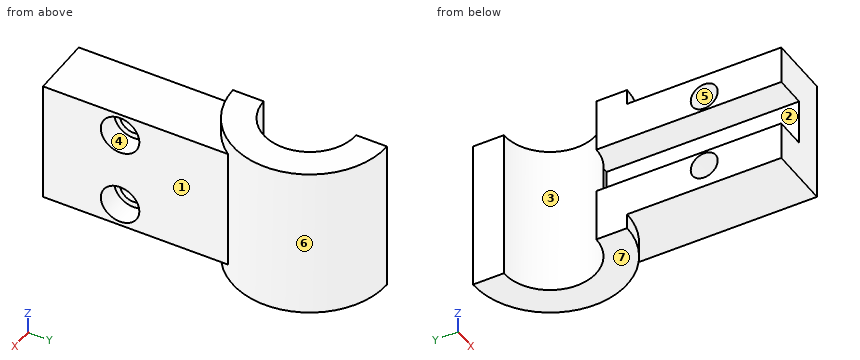
```python
from build123d import *

# Parameters (mm, degrees)
F1_DEPTH = 4
F2_DEPTH = 5
F3_W     = 12
F3_H     = 3
F3_W_2   = 0.4951214439
F4_DEPTH = 2
F5_R     = 1.25
F5_R_2   = 0.875
F6_DEPTH = 1.5
F7_DEPTH = 25


with BuildPart() as f1:
    # F0 (on Top) → F1 (new body, symmetric)
    with BuildSketch(Plane.XY):
        with BuildLine():
            Line((-2.528, 23.2174559587), (1.472, 23.2174559587))
            Line((1.472, 23.2174559587), (1.472, 35.2174559587))
            ThreePointArc((1.472, 35.2174559587), (-0.2919320225, 33.7453200037), (-2.528, 33.2174559587))
            Line((-2.528, 33.2174559587), (-2.528, 23.2174559587))
        make_face()
    extrude(amount=F1_DEPTH, both=True)

    # F0 (on Top) → F2 (join, symmetric)
    with BuildSketch(Plane.XY):
        with BuildLine():
            ThreePointArc((-2.528, 33.2174559587), (-0.2919320225, 33.7453200037), (1.472, 35.2174559587))
            ThreePointArc((1.472, 35.2174559587), (1.944135955, 40.4535239362), (-2.528, 43.2174559587))
            Line((-2.528, 43.2174559587), (-2.528, 41.2174559587))
            ThreePointArc((-2.528, 41.2174559587), (0.472, 38.2174559587), (-2.528, 35.2174559587))
            Line((-2.528, 35.2174559587), (-2.528, 33.2174559587))
        make_face()
    extrude(amount=F2_DEPTH, both=True)

    # F3 (on face) → F4 (cut)
    with BuildSketch(Plane(origin=(-2.528, 0, 0), x_dir=(0, -1, 0), z_dir=(-1, 0, 0))):
        with Locations((-29.2174559587, 0)):
            Rectangle(F3_W, F3_H)
        with Locations((-35.4650166806, 0)):
            Rectangle(F3_W_2, F3_H)
    extrude(amount=-F4_DEPTH, mode=Mode.SUBTRACT)

    # F5 (on face) → F6 (cut)
    with BuildSketch(Plane.YZ.offset(1.472)):
        with Locations((28.2174559587, 2.5)):
            Circle(F5_R)
        with Locations((28.2174559587, 2.5)):
            Circle(F5_R_2, mode=Mode.SUBTRACT)
        with Locations((28.2174559587, -2.5)):
            Circle(F5_R)
        with Locations((28.2174559587, -2.5)):
            Circle(F5_R_2, mode=Mode.SUBTRACT)
    extrude(amount=-F6_DEPTH, mode=Mode.SUBTRACT)

    # F7 (cut): faces of the model
    f7_faces = [f1.faces().sort_by_distance(p)[0] for p in [
        (1.472, 28.2174559587, 2.5),
        (1.472, 28.2174559587, -2.5),
    ]]
    extrude(f7_faces, amount=-F7_DEPTH, mode=Mode.SUBTRACT)


solid = f1.part
```
Part model, mm, in its own coordinate system. Face numbers are marked on the shaded views. A direction names the side the tool comes from. Coordinates: 2 decimals unless noted, no trailing zeros. Order: outer loops, then holes, each group sorted by start corner. A loop starts at its lowest first (then second) coordinate and runs counter-clockwise, first axis right, second up. Notation, with made-up numbers: (63.25, 4) - (80.25, 4) arc R18 cw to (80.25, 18) - close; hole circle Ø10 at (56.5, -14). An arc over 180 degrees is marked (long way). Return JSON: item names as keys, results as strings. Group by question number.
Item 1: Cut at B-B (x = -0.3). List the corners of the cut face in (y, z) (3 decimals).
Item 2: Pin check, flat tips, straight feed: pin 1 (0.9 mm diameter, centred on y = 32.5, z = -0.5, fed in from -X); pin 2 (1.2 mm diameter, centred on x = 0.5, y = 27.5, fed in from +Z); pin 3 (2 mm diameter, centred on x = 1.5, z = -0.5, fed in from +Y). Stop position of each tip, or through.
Item 3: Cut at D-D (x = 1.25). List the corners of the cut face in (y, z), plus the area to 3 significant figures.
Item 4: Cut at A-A (z = 2.5). List the corners of the cut face in (x, y).
Item 5: Pull direction Z, two halves, no side cores. Call the marked faces 5, 6 and 7: pulls with the +Z half, pulls with the -Z half, needs draft (parallel to the pull), parting line crosses it, or undercut.
Item 6: Which spindle directions (+Z, -Z, +X, -X, +Y, -Y) get a long thin tool onto all of the face, cutting with end or side? Do the marked faces 1, 2, 3 and 4. Say none if no direction does.
Item 7: Drill centre lines: probe 1 along Z at (x, y) = (-0.9, 31.25); probe 2 along Y at (x, z) = (-1.65, 3); probe 3 along Y at (x, z) = (-0.1, -3.25). Where is each one in solid material? Low to high. Write a range as from..to.
Item 8: Cut at C-C (z = 1). List the corners of the cut face in (x, y), plus the area to 3 significant figures.
Check values:
{
 "1": {"outline": "(23.217, -4) - (33.741, -4) - (33.741, -5) - (36.208, -5) - (36.208, 5) - (33.741, 5) - (33.741, 4) - (23.217, 4) - close; (40.226, -5) - (42.694, -5) - (42.694, 5) - (40.226, 5) - close; hole circle Ø1.75 at (28.217, -2.5); hole circle Ø1.75 at (28.217, 2.5)"},
 "2": {"pin 1": "stops at x = -0.53", "pin 2": "stops at z = 4", "pin 3": "stops at y = 42.2"},
 "3": {"outline": "(23.22, -4) - (34.94, -4) - (34.94, -5) - (41.49, -5) - (41.49, 5) - (34.94, 5) - (34.94, 4) - (23.22, 4) - close; hole circle Ø2.5 at (28.22, -2.5); hole circle Ø2.5 at (28.22, 2.5)", "area": "149 mm2"},
 "4": {"outline": "(-2.53, 23.22) - (1.47, 23.22) - (1.47, 26.97) - (-0.03, 26.97) - (-0.03, 27.34) - (-2.53, 27.34) - close; (-2.53, 29.09) - (-0.03, 29.09) - (-0.03, 29.47) - (1.47, 29.47) - (1.47, 35.22) arc R5 ccw to (-2.53, 43.22) - (-2.53, 41.22) arc R3 cw to (-2.53, 35.22) - close"},
 "5": {"face 5": "undercut", "face 6": "needs draft", "face 7": "pulls with the -Z half"},
 "6": {"face 1": "+Z, -Z, +X, -Y", "face 2": "-X, -Y", "face 3": "+Z, -Z, -X", "face 4": "+X"},
 "7": {"probe 1": "z = -4..-1.5, 1.5..4", "probe 2": "y = 23.22..27.5, 28.94..35.35, 41.09..43.14", "probe 3": "y = 23.22..27.77, 28.67..36.46, 39.98..42.59"},
 "8": {"outline": "(-2.53, 41.22) arc R3 cw to (-0.88, 35.71) - (-0.53, 35.71) - (-0.53, 23.22) - (1.47, 23.22) - (1.47, 35.22) arc R5 ccw to (-2.53, 43.22) - close", "area": "43.1 mm2"}
}
